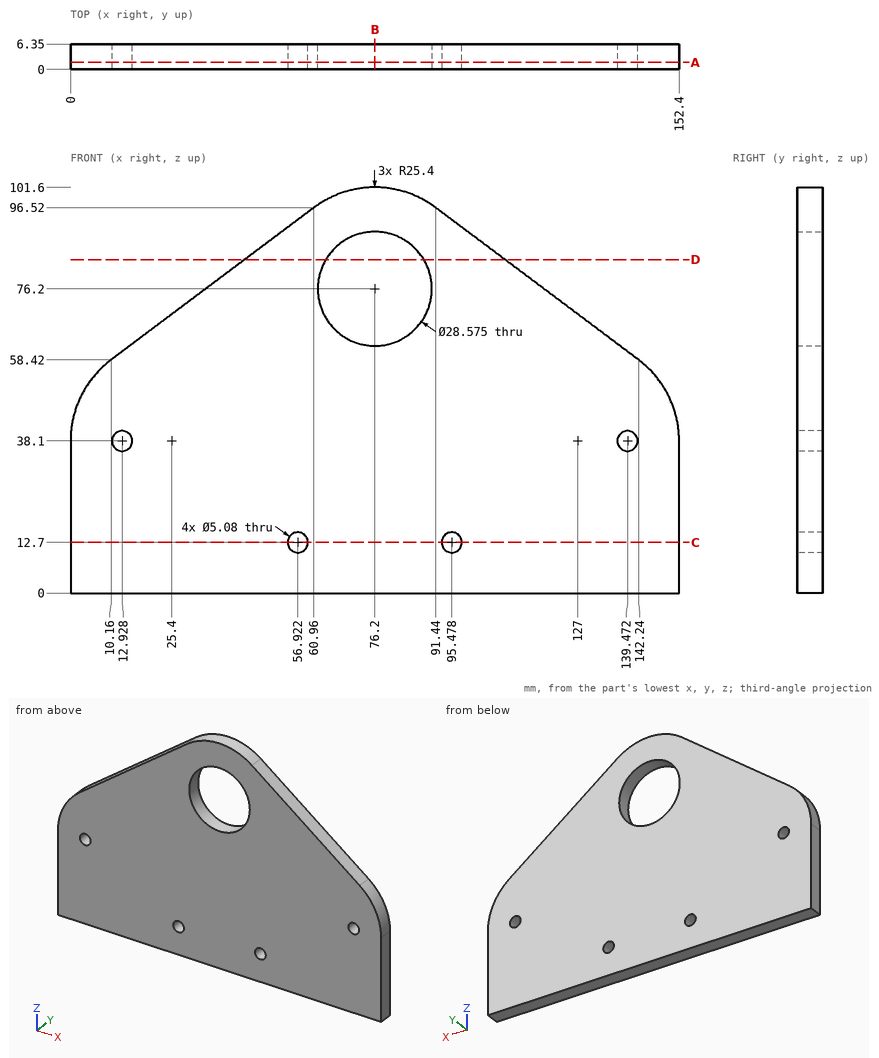
Design review of the part shown in the three views and the two pictorial views. Dimensions are in mm from the part's minimum x, y and z. Round coordinates to 2 decimals unless told otherwise and drop trailing zeros. Loops run counter-clockwise (first coordinate to the right, second up) from the corner with the lowest first, then second, coordinate; pieces in that order, holes last.
Q1. To check wall thickness, follow line 1 along Z through (x, y) = (76.2, 3.5); line 2 along X through (y, z) = (3.25, 14); line 3 along Z through (x, y) = (88, 2.75). State the ranges of each line that lie inside material, in increasing order.
Result sheet:
line 1: z = 0 to 61.91, 90.49 to 101.6
line 2: x = 0 to 54.74, 59.1 to 93.3, 97.66 to 152.4
line 3: z = 0 to 68.14, 84.26 to 98.69
Q2. Add section A-A on y = 1.75. Write out the cut boundary in (x, z) (1 decimal), plus the area to 3 significant figures.
Result sheet:
outline: (0, 0) - (152.4, 0) - (152.4, 38.1) arc R25.4 ccw to (142.2, 58.4) - (91.4, 96.5) arc R25.4 ccw to (61, 96.5) - (10.2, 58.4) arc R25.4 ccw to (0, 38.1) - close; hole circle Ø5.1 at (12.9, 38.1); hole circle Ø5.1 at (56.9, 12.7); hole circle Ø28.6 at (76.2, 76.2); hole circle Ø5.1 at (95.5, 12.7); hole circle Ø5.1 at (139.5, 38.1)
area: 11,300 mm2
Q3. Add section B-B on x = 76.2. Write out the cut boundary in (y, z).
Result sheet:
outline: (0, 0) - (6.35, 0) - (6.35, 61.91) - (0, 61.91) - close; (0, 90.49) - (6.35, 90.49) - (6.35, 101.6) - (0, 101.6) - close
Q4. Insertion check: pin 1 Ø4 at (x, z) = (56.92, 12.7) entering from +Y; pin 2 Ø1.5 at (x, y) = (132, 2.5) entering from +Z. Each pin has a flat end and moves straight along its axis. Give the tip position at first contact, or say it passes through.
Result sheet:
pin 1: passes through
pin 2: stops at z = 66.66
Q5. Add section D-D on z = 83.5. Write out the cut boundary in (x, y), plus the area to 3 significant figures.
Result sheet:
outline: (43.6, 0) - (63.92, 0) - (63.92, 6.35) - (43.6, 6.35) - close; (88.48, 0) - (108.8, 0) - (108.8, 6.35) - (88.48, 6.35) - close
area: 258 mm2
Q6. Add section C-C on z = 12.7. Write out the cut boundary in (x, y), plus the area to 3 significant figures.
Result sheet:
outline: (0, 0) - (54.38, 0) - (54.38, 6.35) - (0, 6.35) - close; (59.46, 0) - (92.94, 0) - (92.94, 6.35) - (59.46, 6.35) - close; (98.02, 0) - (152.4, 0) - (152.4, 6.35) - (98.02, 6.35) - close
area: 903 mm2
